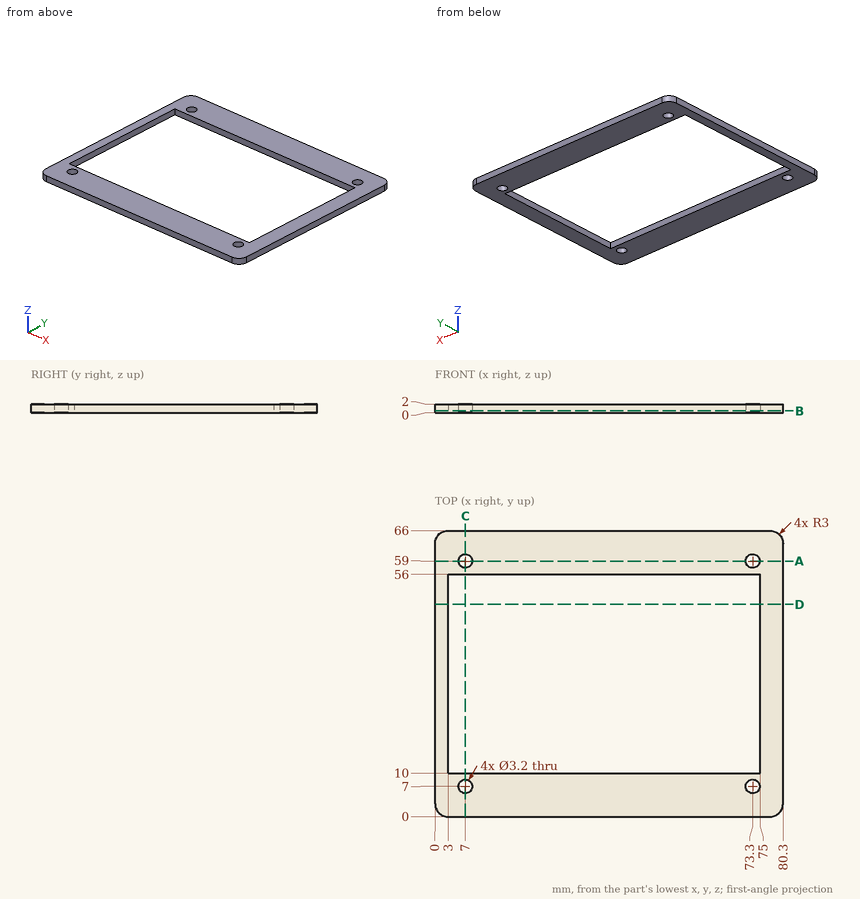
Source: three-view drawing plus pictorial views. Frame: mm from the lowest corner of the part. Coordinates: 2 decimals unless noted, no trailing zeros. Write each loop counter-clockwise with the first axis right and the second up, starting at its lowest first coordinate (ties: lowest second). Pieces come first, ordered by that corner, then holes. Notation, with made-up numbers: (-6.75, -36.75) -> (25.25, -36.75) arc R15 ccw to (25.25, -14.75) -> close; hole circle Ø11 at (40, 65.5). An arc over 180 degrees is marked (long way). Write each question's results on one line, items separated by ' | '.
Item 1: Pin query (flat end, axial travel): pin 1 Ø5 at (x, y) = (7, 59) entering from -Z. Return the tip coordinate at first contact, or that it passes through.
Conclusion:
pin 1: stops at z = 0
Item 2: Section query B-B on z = 0.4. Return loops of the section in (x, y), plus the area to 3 significant figures.
Conclusion:
outline: (0, 3) arc R3 ccw to (3, 0) -> (77.3, 0) arc R3 ccw to (80.3, 3) -> (80.3, 63) arc R3 ccw to (77.3, 66) -> (3, 66) arc R3 ccw to (0, 63) -> close; hole (3, 10) -> (75, 10) -> (75, 56) -> (3, 56) -> close; hole circle Ø3.2 at (7, 7); hole circle Ø3.2 at (7, 59); hole circle Ø3.2 at (73.3, 7); hole circle Ø3.2 at (73.3, 59) | area: 1,950 mm^2
Item 3: Section query A-A on y = 59. Return loops of the section in (x, z).
Conclusion:
outline: (0, 0) -> (5.4, 0) -> (5.4, 2) -> (0, 2) -> close; (8.6, 0) -> (71.7, 0) -> (71.7, 2) -> (8.6, 2) -> close; (74.9, 0) -> (80.3, 0) -> (80.3, 2) -> (74.9, 2) -> close
Item 4: Material intervals for probe 1 along Y at (x, z) = (73.3, 1.45); probe 2 along Y at (x, z) = (15.5, 0.8); probe 3 along X at (y, z) = (17, 1.2), sorted ascending.
Conclusion:
probe 1: y = 0 to 5.4, 8.6 to 10, 56 to 57.4, 60.6 to 66 | probe 2: y = 0 to 10, 56 to 66 | probe 3: x = 0 to 3, 75 to 80.3
Item 5: Section query C-C on x = 7. Return loops of the section in (y, z).
Conclusion:
outline: (0, 0) -> (5.4, 0) -> (5.4, 2) -> (0, 2) -> close; (8.6, 0) -> (10, 0) -> (10, 2) -> (8.6, 2) -> close; (56, 0) -> (57.4, 0) -> (57.4, 2) -> (56, 2) -> close; (60.6, 0) -> (66, 0) -> (66, 2) -> (60.6, 2) -> close
Item 6: Section query D-D on y = 49. Return loops of the section in (x, z).
Conclusion:
outline: (0, 0) -> (3, 0) -> (3, 2) -> (0, 2) -> close; (75, 0) -> (80.3, 0) -> (80.3, 2) -> (75, 2) -> close
